Source: CAD feature listing. Evaluate the final solid. Frame: model axes, mm. A direction names the side the tool comes from. Round coordinates to 2 decimals unless told otherwise and drop trailing zeros. Loops run counter-clockwise (first coordinate to the right, second up) from the corner with the lowest first, then second, coordinate; pieces in that order, holes last. Notation, with made-up numbers: (18, 16) - (66, 16) arc R17 cw to (66, 44) - close; hole circle Ø8 at (11, -35.5). An arc over 180 degrees is marked (long way). Use CSV: the item, a comma, the result in double quotes. Start each with the question number.
from build123d import *

# Parameters (mm, degrees)
SKETCH_2_R               = 7
CUT_EXTRUDE_1_DEPTH      = 13
CUT_EXTRUDE_2_DEPTH      = 18
CUT_EXTRUDE_3_DEPTH      = 35.073450075
CUT_EXTRUDE_3_DEPTH_BACK = 35.073450075
SKETCH_4_R               = 1.5
SKETCH_5_R               = 2
CUT_EXTRUDE_4_DEPTH      = 4
CUT_EXTRUDE_5_DEPTH      = 35.073450166
CUT_EXTRUDE_5_DEPTH_BACK = 35.073450166
SKETCH_6_R               = 1.5


with BuildPart() as part:
    # 草图1 → 旋转1 (revolve)
    with BuildSketch(Plane.XY, mode=Mode.PRIVATE) as revolve_1_sk:
        Polygon((0, 0), (10, 0), (10, 19), (6, 19), (6, 31), (0, 31), align=None)
    revolve(revolve_1_sk.sketch.rotate(Axis((0, 31, 0), (0, -1, 0)), 180), axis=Axis((0, 31, 0), (0, -1, 0)))

    # 草图2 → 切除-拉伸1 (cut)
    with BuildSketch(Plane(origin=(0, 3, 0), x_dir=(1, 0, 0), z_dir=(0, 1, 0))):
        with Locations(Location((0, 0, 0), (0, 0, 90))):
            Circle(SKETCH_2_R)
    extrude(amount=CUT_EXTRUDE_1_DEPTH, mode=Mode.SUBTRACT)

    # 草图3 → 切除-拉伸2 (cut)
    with BuildSketch(Plane.XY):
        Polygon((0, 3), (6, 3), (6, 16), (-6, 16), (-6, 3), align=None)
    extrude(amount=CUT_EXTRUDE_2_DEPTH, mode=Mode.SUBTRACT)

    # 草图4 → 切除-拉伸3 (cut, two sides: drawn at the far end of the back side and taken through both)
    with BuildSketch(Plane.XY.offset(-CUT_EXTRUDE_3_DEPTH_BACK)):
        with Locations((0, 27)):
            Circle(SKETCH_4_R)
    extrude(amount=CUT_EXTRUDE_3_DEPTH + CUT_EXTRUDE_3_DEPTH_BACK, mode=Mode.SUBTRACT)

    # 草图5 → 切除-拉伸4 (cut)
    with BuildSketch(Plane.XZ):
        with Locations(Location((0, 0, 0), (0, 0, 270))):
            Circle(SKETCH_5_R)
    extrude(amount=-CUT_EXTRUDE_4_DEPTH, mode=Mode.SUBTRACT)

    # 草图6 → 切除-拉伸5 (cut, two sides: drawn at the far end of the back side and taken through both)
    with BuildSketch(Plane(origin=(0, 0, 0), x_dir=(0, 0, -1), z_dir=(1, 0, 0)).offset(-CUT_EXTRUDE_5_DEPTH_BACK)):
        with Locations((0, 23)):
            Circle(SKETCH_6_R)
    extrude(amount=CUT_EXTRUDE_5_DEPTH + CUT_EXTRUDE_5_DEPTH_BACK, mode=Mode.SUBTRACT)


solid = part.part
1. Contact query for flat-ended pins moving along their axis: P1, Ø10, axis at y = 14, z = -6, coming from the -X side; P2, Ø1, axis at x = 6.5, y = 13.5, coming from the -Z side; P3, Ø1.5, axis at y = 17.5, z = -1.5, coming from the -X side; P4, Ø1.8, axis at x = 0, y = 27, coming from the +Z side. Output: stop coordinate, or through.
2. Line query: line 1 along Y through (x, z) = (0, 2.75); line 2 along X through (y, z) = (27, 0.25); line 3 along Y through (x, z) = (-3, -0.25). Output: solid intervals per line, ascending.
3. Mould query, pull axis Z, two halves, no side actions, for faces 3 (the cylindrical face through (0, 9, -7)), 4 (the cylindrical face through (-5.54, 25.08, 2.3)), 5 (the cylindrical face through (-2, 1, 0)), 6 (the flat face through (-7, 19, 0)). Classes: +Z half, -Z half, draft (parallel to the pull), parting line (faces both ways), or undercut.
4. Reachability of faces 1 (the flat face through (0, 31, 0)), 2 (the flat face through (6, 9, 6)) from +Z, -Z, +X, -X, +Y, -Y: full face, straight path, thin tool, end or side. Return the list, or none.
5. Section query B-B on x = 0. Return the cut outline in (y, z).
6. Section query D-D on x = -4. Return the cut outline in (y, z).
7. Section query C-C on y = 2. Return the cut outline in (x, z).
8. Section query A-A on z = 0. Return the cut outline in (x, y), and give its area (3 significant figures).
Values:
1,P1,"stops at x = -9.95"
1,P2,"stops at z = -8"
1,P3,"stops at x = -9.97"
1,P4,"passes through"
2,line 1,"y = 0 to 3, 16 to 25.5, 28.5 to 31"
2,line 2,"x = -5.99 to -1.5, 1.5 to 5.99"
2,line 3,"y = 0 to 3, 16 to 21.52, 24.48 to 31"
3,face 3,"undercut"
3,face 4,"parting line"
3,face 5,"undercut"
3,face 6,"draft"
4,face 1,"+Z, -Z, +X, -X, +Y"
4,face 2,"+Z"
5,outline,"(0, -10) - (19, -10) - (19, -6) - (25.5, -6) - (25.5, 6) - (19, 6) - (19, 10) - (16, 10) - (16, -7) - (3, -7) - (3, -2) - (0, -2) - close; (0, 2) - (3, 2) - (3, 10) - (0, 10) - close; (28.5, -6) - (31, -6) - (31, 6) - (28.5, 6) - close; hole circle Ø3 at (23, 0)"
6,outline,"(0, -9.17) - (19, -9.17) - (19, -4.47) - (31, -4.47) - (31, 4.47) - (19, 4.47) - (19, 9.17) - (16, 9.17) - (16, -5.74) - (3, -5.74) - (3, 9.17) - (0, 9.17) - close; hole circle Ø3 at (23, 0)"
7,outline,"circle Ø20 at (0, 0); hole circle Ø4 at (0, 0)"
8,outline,"(-10, 0) - (-2, 0) - (-2, 3) - (-7, 3) - (-7, 16) - (7, 16) - (7, 3) - (2, 3) - (2, 0) - (10, 0) - (10, 19) - (6, 19) - (6, 21.5) - (-6, 21.5) - (-6, 19) - (-10, 19) - close; (-6, 24.5) - (6, 24.5) - (6, 31) - (-6, 31) - close; hole circle Ø3 at (0, 27)"
8,area,"287 mm^2"
